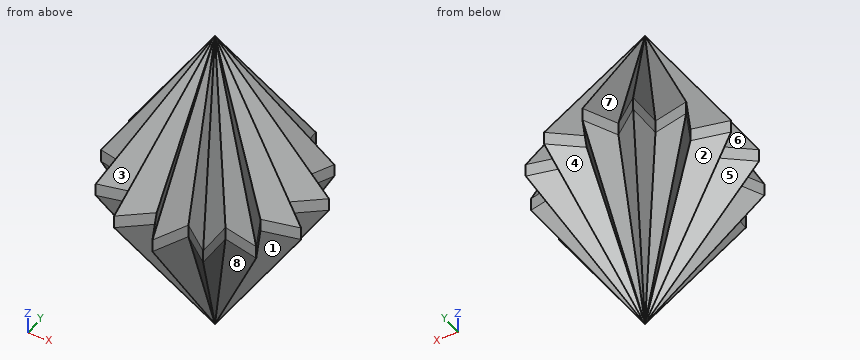
```python
from build123d import *

# Parameters (mm, degrees)
F2_DEPTH = 2


with BuildPart() as f2:
    # F0 (on Top) → F2 (new body)
    with BuildSketch(Plane.XY):
        Polygon((-13.892356, 11.078785), (-17.323485, -3.953972), (-7.709676, -16.009307), (7.709676, -16.009307), (17.323485, -3.953972), (13.892356, 11.078785), (0, 17.768991), (-13.897051, 28.857524), align=None)
        Polygon((17.323485, -3.953972), (7.709676, -16.009307), (25.041621, -19.970026), align=None)
        Polygon((13.892356, 11.078785), (17.323485, -3.953972), (31.226391, 7.12722), align=None)
        Polygon((7.709676, -16.009307), (-7.709676, -16.009307), (0, -32.029435), align=None)
        Polygon((-7.709676, -16.009307), (-17.323485, -3.953972), (-25.041621, -19.970026), align=None)
        Polygon((-31.226391, 7.12722), (-17.323485, -3.953972), (-13.892356, 11.078785), align=None)
        Polygon((13.897051, 28.857524), (0, 17.768991), (13.892356, 11.078785), align=None)
    extrude(amount=F2_DEPTH)

    # F2_face (on face) → F4 section 0
    with BuildSketch(Plane.XY.offset(2), mode=Mode.PRIVATE) as f4_s0:
        Polygon((0, 17.768991), (-13.897051, 28.857524), (-13.892356, 11.078785), (-31.226391, 7.12722), (-17.323485, -3.953972), (-25.041621, -19.970026), (-7.709676, -16.009307), (0, -32.029435), (7.709676, -16.009307), (25.041621, -19.970026), (17.323485, -3.953972), (31.226391, 7.12722), (13.892356, 11.078785), (13.897051, 28.857524), align=None)
    loft([Vertex(0, 0, 50), f4_s0.sketch])

    # F5: F2 across face


with BuildPart() as f2_1:
    add(f2.part)
    add(f2.part.mirror(Plane(origin=(0, 0, 0), x_dir=(1, 0, 0), z_dir=(0, 0, -1))))

    # F6: F2 across plane


with BuildPart() as f2_2:
    add(f2_1.part)
    add(f2_1.part.mirror(Plane.XZ))


solid = f2_2.part
```
The model under review builds one solid part; all positions refer to its coordinate system, in mm. Face numbers are marked on the shaded views. A direction names the side the tool comes from. Round coordinates to 2 decimals unless told otherwise and drop trailing zeros. Order: outer loops, then holes, each group sorted by start corner. A loop starts at its lowest first (then second) coordinate and runs counter-clockwise, first axis right, second up.
(1) Take a section at D-D, the plane x = -26.5. State the section outline as (y, z) points.
Working result:
outline: (-8.2, -2) - (-6.05, -9.27) - (-3.36, -2) - (-3.36, 2) - (-6.05, 9.27) - (-8.2, 2) - close; (3.36, -2) - (6.05, -9.27) - (8.2, -2) - (8.2, 2) - (6.05, 9.27) - (3.36, 2) - close
(2) Take a section at A-A, the plane y = -27.5. State the section outline as (x, z) points.
Working result:
outline: (-13.9, -2) - (-13.24, -4.26) - (-12.2, -2) - (-12.2, 2) - (-13.24, 4.26) - (-13.9, 2) - close; (-2.18, -2) - (0, -8.79) - (2.18, -2) - (2.18, 2) - (0, 8.79) - (-2.18, 2) - close; (12.2, -2) - (13.24, -4.26) - (13.9, -2) - (13.9, 2) - (13.24, 4.26) - (12.2, 2) - close
(3) Wall thickness on L1, parallel to X at y = -16.5, z = -21; L2, parallel to X at y = -19.5, z = -8.5; L3, parallel to Y at x = -19.5, z = -18: over which ranges is each line inside the solid? List them lowest first.
Working result:
L1: x = -8.4 to -7.22, -1.37 to 1.37, 7.22 to 8.4
L2: x = -12.01 to -5.19, -3.94 to 3.94, 5.19 to 12.01
L3: y = -5.05 to -3.7, 3.7 to 5.05
(4) Mouldability with a two-part tool opening along X and no side actions: class the marked faces 1, 2 and 3 as released by +X, released by -X, zero draft, split by the parting line, or undercut.
Working result:
face 1: released by +X
face 2: released by -X
face 3: undercut
(5) For P1, Ø6, axis at y = 20, z = 22, coming from the -X side; P2, Ø2, axis at y = -9.5, z = -20.5, coming from the +X side; P3, Ø5, axis at y = 3, z = -9.5, coming from the +X side, all flat-tipped, find the tip position at first contact; note any pin that passes through.
Working result:
P1: stops at x = -8.83
P2: stops at x = 14.63
P3: stops at x = 25.91
(6) Tool access review of the marked faces 4, 5, 6, 7 and 8: name each direction out of +Z, -Z, +X, -X, +Y, -Y from which nothing blocks a thin tool from reaching the whole face with its end or side.
Working result:
face 4: -Z, +Y
face 5: -Z, -X
face 6: +Z, -X
face 7: +Z, +Y
face 8: -Z, -Y
(7) Take a section at C-C, the plane z = -38.5. State the section outline as (x, y) points.
Working result:
outline: (-7.48, -1.71) - (-4.81, -2.32) - (-6, -4.78) - (-3.33, -4.17) - (-3.33, -6.91) - (-1.19, -5.21) - (0, -7.67) - (1.19, -5.21) - (3.33, -6.91) - (3.33, -4.17) - (6, -4.78) - (4.81, -2.32) - (7.48, -1.71) - (5.34, 0) - (7.48, 1.71) - (4.81, 2.32) - (6, 4.78) - (3.33, 4.17) - (3.33, 6.91) - (1.19, 5.21) - (0, 7.67) - (-1.19, 5.21) - (-3.33, 6.91) - (-3.33, 4.17) - (-6, 4.78) - (-4.81, 2.32) - (-7.48, 1.71) - (-5.34, 0) - close
